```python
from build123d import *

# Parameters (mm, degrees)
EXTRUDE_1_DEPTH     = 3
SKETCH_6_R          = 2
SKETCH_6_R_2        = 2.05
CUT_EXTRUDE_2_DEPTH = 3


with BuildPart() as part:
    # 草图1 → 凸台-拉伸1 (new body)
    with BuildSketch(Plane(origin=(0, 0, 0), x_dir=(1, 0, 0), z_dir=(0, 1, 0))):
        Polygon((-268, 178.5), (-268, -178.5), (-146, -178.5), (-146, -129), (146, -129), (146, -178.5), (268, -178.5), (268, 178.5), (146, 178.5), (146, 129), (-146, 129), (-146, 178.5), align=None)
    extrude(amount=EXTRUDE_1_DEPTH)

    # 草图6 → 切除-拉伸2 (cut)
    with BuildSketch(Plane.XZ):
        with Locations(Location((172, 175.5, 0), (0, 0, 270))):
            Circle(SKETCH_6_R)
        with Locations(Location((242, 175.5, 0), (0, 0, 270))):
            Circle(SKETCH_6_R)
        with Locations(Location((170.5, 151, 0), (0, 0, 270))):
            Circle(SKETCH_6_R_2)
        with Locations(Location((192.5, 151, 0), (0, 0, 270))):
            Circle(SKETCH_6_R_2)
        with Locations(Location((192.5, 141, 0), (0, 0, 270))):
            Circle(SKETCH_6_R_2)
        with Locations(Location((170.5, 141, 0), (0, 0, 270))):
            Circle(SKETCH_6_R_2)
        with Locations(Location((221.5, 151, 0), (0, 0, 270))):
            Circle(SKETCH_6_R_2)
        with Locations(Location((221.5, 141, 0), (0, 0, 270))):
            Circle(SKETCH_6_R_2)
        with Locations(Location((243.5, 151, 0), (0, 0, 270))):
            Circle(SKETCH_6_R_2)
        with Locations(Location((243.5, 141, 0), (0, 0, 270))):
            Circle(SKETCH_6_R_2)
        with Locations(Location((172, 50.5, 0), (0, 0, 270))):
            Circle(SKETCH_6_R)
        with Locations(Location((242, 50.5, 0), (0, 0, 270))):
            Circle(SKETCH_6_R)
        with Locations(Location((100, 126, 0), (0, 0, 270))):
            Circle(SKETCH_6_R)
        with Locations(Location((120, 126, 0), (0, 0, 270))):
            Circle(SKETCH_6_R)
        with Locations(Location((242, -50.5, 0), (0, 0, 90))):
            Circle(SKETCH_6_R)
        with Locations(Location((172, -50.5, 0), (0, 0, 90))):
            Circle(SKETCH_6_R)
        with Locations(Location((243.5, -141, 0), (0, 0, 90))):
            Circle(SKETCH_6_R_2)
        with Locations(Location((243.5, -151, 0), (0, 0, 90))):
            Circle(SKETCH_6_R_2)
        with Locations(Location((221.5, -141, 0), (0, 0, 90))):
            Circle(SKETCH_6_R_2)
        with Locations(Location((221.5, -151, 0), (0, 0, 90))):
            Circle(SKETCH_6_R_2)
        with Locations(Location((192.5, -141, 0), (0, 0, 90))):
            Circle(SKETCH_6_R_2)
        with Locations(Location((170.5, -141, 0), (0, 0, 90))):
            Circle(SKETCH_6_R_2)
        with Locations(Location((170.5, -151, 0), (0, 0, 90))):
            Circle(SKETCH_6_R_2)
        with Locations(Location((192.5, -151, 0), (0, 0, 90))):
            Circle(SKETCH_6_R_2)
        with Locations(Location((242, -175.5, 0), (0, 0, 90))):
            Circle(SKETCH_6_R)
        with Locations(Location((172, -175.5, 0), (0, 0, 90))):
            Circle(SKETCH_6_R)
        with Locations(Location((120, -126, 0), (0, 0, 90))):
            Circle(SKETCH_6_R)
        with Locations(Location((100, -126, 0), (0, 0, 90))):
            Circle(SKETCH_6_R)
        with Locations(Location((-172, -175.5, 0), (0, 0, 270))):
            Circle(SKETCH_6_R)
        with Locations(Location((-242, -175.5, 0), (0, 0, 270))):
            Circle(SKETCH_6_R)
        with Locations(Location((-221.5, -151, 0), (0, 0, 270))):
            Circle(SKETCH_6_R_2)
        with Locations(Location((-243.5, -151, 0), (0, 0, 270))):
            Circle(SKETCH_6_R_2)
        with Locations(Location((-243.5, -141, 0), (0, 0, 270))):
            Circle(SKETCH_6_R_2)
        with Locations(Location((-221.5, -141, 0), (0, 0, 270))):
            Circle(SKETCH_6_R_2)
        with Locations(Location((-170.5, -151, 0), (0, 0, 270))):
            Circle(SKETCH_6_R_2)
        with Locations(Location((-192.5, -151, 0), (0, 0, 270))):
            Circle(SKETCH_6_R_2)
        with Locations(Location((-192.5, -141, 0), (0, 0, 270))):
            Circle(SKETCH_6_R_2)
        with Locations(Location((-170.5, -141, 0), (0, 0, 270))):
            Circle(SKETCH_6_R_2)
        with Locations(Location((-100, -126, 0), (0, 0, 270))):
            Circle(SKETCH_6_R)
        with Locations(Location((-120, -126, 0), (0, 0, 270))):
            Circle(SKETCH_6_R)
        with Locations(Location((-242, -50.5, 0), (0, 0, 270))):
            Circle(SKETCH_6_R)
        with Locations(Location((-172, -50.5, 0), (0, 0, 270))):
            Circle(SKETCH_6_R)
        with Locations(Location((-242, 50.5, 0), (0, 0, 90))):
            Circle(SKETCH_6_R)
        with Locations(Location((-172, 50.5, 0), (0, 0, 90))):
            Circle(SKETCH_6_R)
        with Locations(Location((-243.5, 141, 0), (0, 0, 90))):
            Circle(SKETCH_6_R_2)
        with Locations(Location((-243.5, 151, 0), (0, 0, 90))):
            Circle(SKETCH_6_R_2)
        with Locations(Location((-221.5, 141, 0), (0, 0, 90))):
            Circle(SKETCH_6_R_2)
        with Locations(Location((-221.5, 151, 0), (0, 0, 90))):
            Circle(SKETCH_6_R_2)
        with Locations(Location((-192.5, 141, 0), (0, 0, 90))):
            Circle(SKETCH_6_R_2)
        with Locations(Location((-170.5, 141, 0), (0, 0, 90))):
            Circle(SKETCH_6_R_2)
        with Locations(Location((-192.5, 151, 0), (0, 0, 90))):
            Circle(SKETCH_6_R_2)
        with Locations(Location((-170.5, 151, 0), (0, 0, 90))):
            Circle(SKETCH_6_R_2)
        with Locations(Location((-242, 175.5, 0), (0, 0, 90))):
            Circle(SKETCH_6_R)
        with Locations(Location((-172, 175.5, 0), (0, 0, 90))):
            Circle(SKETCH_6_R)
        with Locations(Location((-120, 126, 0), (0, 0, 90))):
            Circle(SKETCH_6_R)
        with Locations(Location((-100, 126, 0), (0, 0, 90))):
            Circle(SKETCH_6_R)
    extrude(amount=-CUT_EXTRUDE_2_DEPTH, mode=Mode.SUBTRACT)


solid = part.part
```
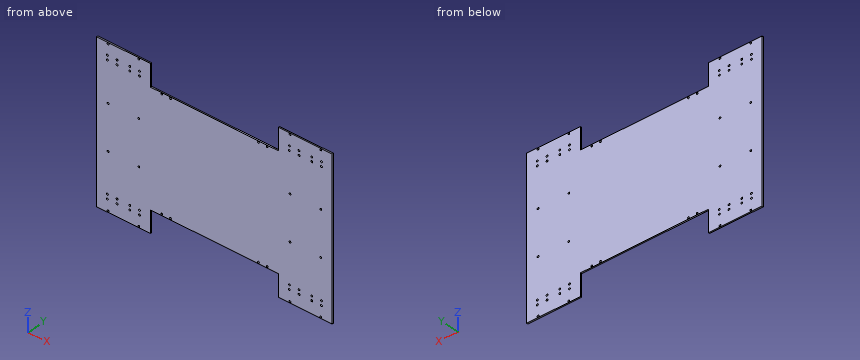
Here's how the part is built. I have some questions about the finished solid (model axes, mm). Round coordinates to 2 decimals unless told otherwise and drop trailing zeros. Order: outer loops, then holes, each group sorted by start corner. A loop starts at its lowest first (then second) coordinate and runs counter-clockwise, first axis right, second up. Notation, with made-up numbers: M 56,16.5 L 96,16.5 A18 ccw 96,45.5 Z; hole C -36.5,-0.75 d6. An arc over 180 degrees is marked long. Answer as CSV lines item,"result".
Item 1: Imagine slicing it at B-B on x = -60.5. List the corners of the cut face in (y, z) for me.
From the geometry:
outline,"M 0,-129 L 3,-129 L 3,129 L 0,129 Z"
Item 2: Imagine slicing it at A-A on y = 0.8. Give the number of separate pieces and of enclosed holes in the cut face, and give its area (3 significant figures).
From the geometry:
separate pieces,"1"
enclosed holes,"56"
area,"162,000 mm2"
Item 3: For pin 1 (2.5 mm diameter, centred on x = 170.5, z = -141, fed in from +Y); pin 2 (6.5 mm diameter, centred on x = 170.5, z = 141, fed in from -Y); pin 3 (1.5 mm diameter, centred on x = -107, y = 2.5, fed in from -Z), each with a flat end and sliding along its axis, tell me the tip position at first contact or that it passes through.
From the geometry:
pin 1,"through"
pin 2,"y = 0"
pin 3,"z = -129"
Item 4: Please list where these lines run through material, in increasing order: L1, parallel to X at y = 1.45, z = -50.5; L2, parallel to X at y = 1.55, z = 175.5; L3, parallel to X at y = 0.1, z = 137.5. Write a range as [from, to].
From the geometry:
L1,"[-268, -244], [-240, -174], [-170, 170], [174, 240], [244, 268]"
L2,"[-268, -244], [-240, -174], [-170, -146], [146, 170], [174, 240], [244, 268]"
L3,"[-268, -146], [146, 268]"
